from build123d import *

# Parameters (mm, degrees)
F0_W      = 52.5
F0_H      = 47.5
F0_R      = 1.75
F0_R_2    = 12.5
F1_DEPTH  = 5
F3_DEPTH  = 25
F4_W      = 52.5
F4_H      = 5
F5_DEPTH  = 20
F7_DEPTH  = 5
F9_DEPTH  = 52.5
F10_R     = 2.75
F11_DEPTH = 30.001
F13_DEPTH = 52.5


with BuildPart() as f1:
    # F0 (on Front) → F1 (new body)
    with BuildSketch(Plane.XZ):
        with Locations((26.25, 23.75)):
            Rectangle(F0_W, F0_H)
        with Locations((10.75, 5.75)):
            Circle(F0_R, mode=Mode.SUBTRACT)
        with Locations((41.75, 5.75)):
            Circle(F0_R, mode=Mode.SUBTRACT)
        with Locations((26.25, 21.25)):
            Circle(F0_R_2, mode=Mode.SUBTRACT)
        with Locations((10.75, 36.75)):
            Circle(F0_R, mode=Mode.SUBTRACT)
        with Locations((41.75, 36.75)):
            Circle(F0_R, mode=Mode.SUBTRACT)
    extrude(amount=F1_DEPTH)

    # F2 (on face) → F3 (join)
    with BuildSketch(Plane.XZ.offset(5)):
        Polygon((0, 47.5), (0, 0), (5, 0), (5, 42.5), (47.5, 42.5), (47.5, 0), (52.5, 0), (52.5, 47.5), align=None)
    extrude(amount=F3_DEPTH)

    # F4 (on face) → F5 (join)
    with BuildSketch(Plane.XY.offset(47.5)):
        with Locations((26.25, -2.5)):
            Rectangle(F4_W, F4_H)
    extrude(amount=F5_DEPTH)

    # F6 (on face) → F7 (join)
    with BuildSketch(Plane.XY.offset(47.5)):
        with BuildLine():
            Line((0, 0), (-14.516609, -12.395098))
            ThreePointArc((-14.516609, -12.395098), (-17.405253, -23.460562), (-8.023115, -30))
            Line((-8.023115, -30), (0, -30))
            Line((0, -30), (0, 0))
        make_face()
        with BuildLine():
            ThreePointArc((-8.023115, -17.25), (-6.078571, -18.055456), (-5.273115, -20))
            ThreePointArc((-5.273115, -20), (-6.078571, -21.944544), (-8.023115, -22.75))
            ThreePointArc((-8.023115, -22.75), (-10.773115, -20), (-8.023115, -17.25))
        make_face(mode=Mode.SUBTRACT)
        with BuildLine():
            ThreePointArc((60.523115, -30), (69.905253, -23.460562), (67.016609, -12.395098))
            Line((67.016609, -12.395098), (52.5, 0))
            Line((52.5, 0), (52.5, -30))
            Line((52.5, -30), (60.523115, -30))
        make_face()
        with BuildLine():
            ThreePointArc((60.523115, -22.75), (57.773115, -20), (60.523115, -17.25))
            ThreePointArc((60.523115, -17.25), (62.467659, -18.055456), (63.273115, -20))
            ThreePointArc((63.273115, -20), (62.467659, -21.944544), (60.523115, -22.75))
        make_face(mode=Mode.SUBTRACT)
    extrude(amount=-F7_DEPTH)

    # F8 (on face) → F9 (join, through all)
    with BuildSketch(Plane.YZ.offset(52.5)):
        Polygon((-6.785, 54.66), (-5, 52.875), (-5, 62.125), (-6.785, 60.34), align=None)
    extrude(amount=-F9_DEPTH)

    # F10 (on face) → F11 (cut, through all)
    with BuildSketch(Plane(origin=(0, 0, 0), x_dir=(-1, 0, 0), z_dir=(0, 1, 0))):
        with Locations((-41.75, 57.5)):
            Circle(F10_R)
        with Locations((-10.75, 57.5)):
            Circle(F10_R)
    extrude(amount=-F11_DEPTH, mode=Mode.SUBTRACT)

    # F12 (on face) → F13 (cut, through all)
    with BuildSketch(Plane.YZ.offset(52.5)):
        Polygon((-5, 0), (-30, 42.5), (-30, 0), align=None)
    extrude(amount=-F13_DEPTH, mode=Mode.SUBTRACT)


solid = f1.part
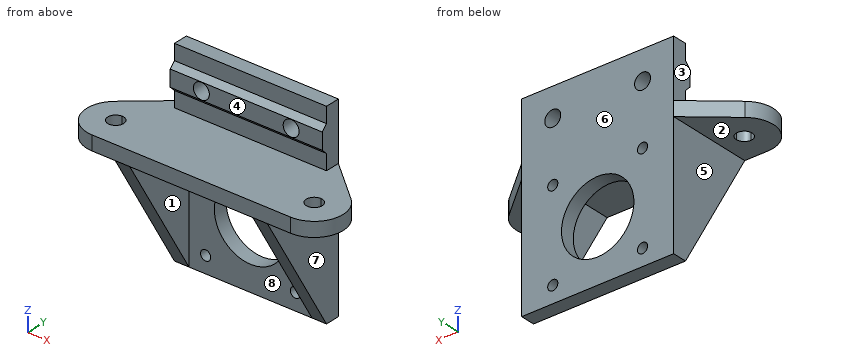
Model file for the job. Use its own axes, mm. Face numbers are marked on the shaded views. A direction names the side the tool comes from. Give positions to 0.01 mm unless a question says otherwise; leave off trailing zeros. Loops run counter-clockwise (first coordinate to the right, second up) from the corner with the lowest first, then second, coordinate; pieces in that order, holes last.
1) Saw through at B-B (z = 57.5). Write the cut outline in (x, y) (3 decimals).
2) Pull direction X, two halves, no side cores. Call the marked faces 5, 6, 7 and 8: +X half, -X half, draft (parallel to the pull), parting line (faces both ways), or undercut.
3) Tool access for the marked faces 1, 2, 3 and 4: list every direction of +Z, -Z, +X, -X, +Y, -Y with a clear straight run to the whole face (end or side of a thin tool).
4) Flat gauge pins, fed straight in: pin 1 Ø2.5 at (x, z) = (25.5, 65.5) entering from -Y; pin 2 Ø2 at (y, z) = (-4.5, 54.5) entering from +X; pin 3 Ø3 at (x, y) = (48.5, -22.5) entering from +Z; pin 4 Ø2 at (x, z) = (10.75, 5.75) entering from +Y. Where does each tip first touch, or does it go through?
5) Saw through at D-D (x = 25). Write the cut outline in (y, z) (3 decimals).
6) Wall check: line 1 (Z direction, x = 41.75, y = -1.75); line 2 (X direction, y = -9.5, z = 19.5); line 3 (X direction, y = -19.5, z = 43). Give the ranges that are in metal, low to high.
7) Saw through at C-C (z = 21.25). Write the cut outline in (x, y), plus the area to 4 significant figures.
8) Saw through at A-A (x = 41.75). Write the cut outline in (y, z) (3 decimals), plus the area to 3 significant figures.
Answer block:
1. outline: (0, -6.785) - (8, -6.785) - (8, 0) - (0, 0) - close; (13.5, -6.785) - (39, -6.785) - (39, 0) - (13.5, 0) - close; (44.5, -6.785) - (52.5, -6.785) - (52.5, 0) - (44.5, 0) - close
2. face 5: -X half
2. face 6: draft
2. face 7: +X half
2. face 8: undercut
3. face 1: -Z, -Y
3. face 2: -Z, -X, +Y, -Y
3. face 3: +Z, -X, +Y, -Y
3. face 4: +Z, +X, -X, -Y
4. pin 1: stops at y = -5
4. pin 2: stops at x = 52.5
4. pin 3: stops at z = 47.5
4. pin 4: passes through
5. outline: (-30, 42.5) - (-5, 42.5) - (-5, 33.687) - (0, 33.687) - (0, 67.5) - (-5, 67.5) - (-5, 62.125) - (-6.785, 60.34) - (-6.785, 54.66) - (-5, 52.875) - (-5, 47.5) - (-30, 47.5) - close; (-5, 0) - (0, 0) - (0, 8.813) - (-5, 8.813) - close
6. line 1: z = 0 to 4, 7.5 to 35, 38.5 to 54.75, 60.25 to 67.5
6. line 2: x = 0 to 5, 47.5 to 52.5
6. line 3: x = -18.01 to -10.73, -5.32 to 57.82, 63.23 to 70.51
7. outline: (0, -17.5) - (5, -17.5) - (5, -5) - (13.75, -5) - (13.75, 0) - (0, 0) - close; (38.75, -5) - (47.5, -5) - (47.5, -17.5) - (52.5, -17.5) - (52.5, 0) - (38.75, 0) - close
7. area: 262.5 mm2
8. outline: (-30, 42.5) - (-5, 42.5) - (-5, 38.5) - (0, 38.5) - (0, 54.75) - (-6.785, 54.75) - (-6.785, 54.66) - (-5, 52.875) - (-5, 47.5) - (-30, 47.5) - close; (-6.785, 60.25) - (0, 60.25) - (0, 67.5) - (-5, 67.5) - (-5, 62.125) - (-6.785, 60.34) - close; (-5, 0) - (0, 0) - (0, 4) - (-5, 4) - close; (-5, 7.5) - (0, 7.5) - (0, 35) - (-5, 35) - close
8. area: 404 mm2
